Can you work these out from the model? Positions are in its coordinate system, mm. Face numbers are marked on the shaded views. A direction names the side the tool comes from. Give positions to 0.01 mm unless a question says otherwise; leave off trailing zeros. Order: outer loops, then holes, each group sorted by start corner. A loop starts at its lowest first (then second) coordinate and runs counter-clockwise, first axis right, second up. Notation, with made-up numbers: (-3, 23) -> (56, 23) arc R25 ccw to (56, 60) -> close; hole circle Ø6 at (61, 16.25). An arc over 180 degrees is marked (long way). Answer as a JSON object with one key per item and string values.
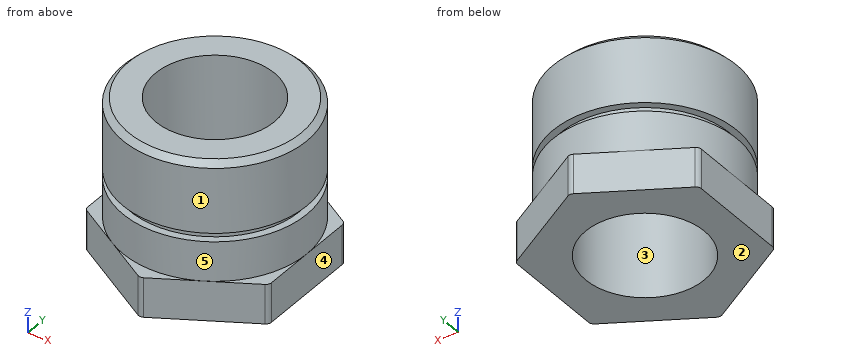
```python
from build123d import *

# Parameters (mm, degrees)
SKETCH1_R           = 32.5
BOSS_EXTRUDE1_DEPTH = 42
CUT_EXTRUDE1_START  = -28
SKETCH2_R           = 32.5
SKETCH2_R_2         = 30
CUT_EXTRUDE1_DEPTH  = 3
BOSS_EXTRUDE3_DEPTH = 14
FILLET1_R           = 2
CHAMFER1_SIZE       = 2
SKETCH4_R           = 21
CUT_EXTRUDE4_DEPTH  = 57


with BuildPart() as part:
    # Sketch1 → Boss-Extrude1 (new body)
    with BuildSketch(Plane.XY):
        Circle(SKETCH1_R)
    extrude(amount=BOSS_EXTRUDE1_DEPTH)

    # Sketch2 → Cut-Extrude1 (cut)
    with BuildSketch(Plane.XY.offset(42).offset(CUT_EXTRUDE1_START)):
        Circle(SKETCH2_R)
        Circle(SKETCH2_R_2, mode=Mode.SUBTRACT)
    extrude(amount=CUT_EXTRUDE1_DEPTH, mode=Mode.SUBTRACT)

    # Sketch3 → Boss-Extrude3 (add)
    with BuildSketch(Plane(origin=(0, 0, 0), x_dir=(-1, 0, 0), z_dir=(0, 0, -1))):
        Polygon((32.5, -18.763883749), (32.5, 18.763883749), (0, 37.527767497), (-32.5, 18.763883749), (-32.5, -18.763883749), (0, -37.527767497), align=None)
    extrude(amount=BOSS_EXTRUDE3_DEPTH)

    # Fillet1
    fillet1_edges = [part.edges().sort_by_distance(p)[0] for p in [
        (0, -37.527767497, -7),
        (-32.5, -18.763883749, -7),
        (-32.5, 18.763883749, -7),
        (0, 37.527767497, -7),
        (32.5, 18.763883749, -7),
        (32.5, -18.763883749, -7),
    ]]
    fillet(fillet1_edges, radius=FILLET1_R)

    # Chamfer1
    chamfer1_edges = [part.edges().sort_by_distance(p)[0] for p in [
        (-32.5, 0, 42),
    ]]
    chamfer(chamfer1_edges, length=CHAMFER1_SIZE)

    # Sketch4 → Cut-Extrude4 (cut, through all)
    with BuildSketch(Plane.XY.offset(42)):
        Circle(SKETCH4_R)
    extrude(amount=-CUT_EXTRUDE4_DEPTH, mode=Mode.SUBTRACT)


solid = part.part
```
1. If we mould it in two halves opening along Y, with no side actions, what happens to the marked faces 3, 4 and 5? For each: +Y half, -Y half, draft (parallel to the pull), parting line (faces both ways), or undercut.
Worked answers:
{"face 3": "undercut", "face 4": "draft", "face 5": "parting line"}
2. If we section it at C-C on z = 28: Please give me the cut outline in (x, y), then the cut area to 3 significant figures.
Worked answers:
{"outline": "circle Ø65 at (0, 0); hole circle Ø42 at (0, 0)", "area": "1,930 mm²"}
3. If we section it at B-B on z = -5: Please give me the cut outline in (x, y), then the cut area to 3 significant figures.
Worked answers:
{"outline": "(-32.5, -17.61) arc R2 ccw to (-31.5, -19.34) -> (-1, -36.95) arc R2 ccw to (1, -36.95) -> (31.5, -19.34) arc R2 ccw to (32.5, -17.61) -> (32.5, 17.61) arc R2 ccw to (31.5, 19.34) -> (1, 36.95) arc R2 ccw to (-1, 36.95) -> (-31.5, 19.34) arc R2 ccw to (-32.5, 17.61) -> close; hole circle Ø42 at (0, 0)", "area": "2,270 mm²"}
4. For the marked faces 1 and 2, which set-ups out of +Z, -Z, +X, -X, +Y, -Y let a thin tool reach every point of the face, with its end or its side?
Worked answers:
{"face 1": "+Z", "face 2": "-Z, +X, -X, +Y, -Y"}
5. Please list where these lines run through material, in increasing order: L1, parallel to Y at x = 0, z = 20; L2, parallel to Y at x = 0, z = 14.5; L3, parallel to X at y = -8, z = 10.
Worked answers:
{"L1": "-32.5 to -21, 21 to 32.5", "L2": "-30 to -21, 21 to 30", "L3": "-31.5 to -19.42, 19.42 to 31.5"}
6. Will these pins go through, and if not, where does the flat tip stop? pin 1 Ø8 at (x, y) = (-28.5, -21) entering from +Z; pin 2 Ø4.5 at (x, y) = (-7.5, 33.5) entering from +Z; pin 3 Ø8 at (x, z) = (-7, 29) entering from +Y.
Worked answers:
{"pin 1": "z = 41.1", "pin 2": "z = 40.42", "pin 3": "y = 32.36"}
7. If we section it at A-A on x = 0: Please give me the cut outline in (y, z).
Worked answers:
{"outline": "(-37.22, -14) -> (-21, -14) -> (-21, 42) -> (-30.5, 42) -> (-32.5, 40) -> (-32.5, 17) -> (-30, 17) -> (-30, 14) -> (-32.5, 14) -> (-32.5, 0) -> (-37.22, 0) -> close; (21, -14) -> (37.22, -14) -> (37.22, 0) -> (32.5, 0) -> (32.5, 14) -> (30, 14) -> (30, 17) -> (32.5, 17) -> (32.5, 40) -> (30.5, 42) -> (21, 42) -> close"}
